Could you check a few things on this model? Use its own coordinates, in mm. A direction names the side the tool comes from. Round coordinates to 2 decimals unless told otherwise and drop trailing zeros. Loops run counter-clockwise (first coordinate to the right, second up) from the corner with the lowest first, then second, coordinate; pieces in that order, holes last. Notation, with made-up numbers: (25.5, -35) -> (65.5, -35) arc R16 cw to (65.5, -9) -> close; hole circle Ø2 at (36.25, -8.5). An arc over 180 degrees is marked (long way). Write each question's results on one line, items separated by ' | '.
Autodesk Inventor part; units mm, degrees
ref_plane "YZ Plane" through (0, 0, 0) normal (1, 0, 0) x (0, 1, 0)
ref_plane "XZ Plane" through (0, 0, 0) normal (0, 1, 0) x (-1, 0, 0)
ref_plane "XY Plane" through (0, 0, 0) normal (0, 0, 1) x (1, 0, 0)
sketch "Sketch1" plane through (0, 0, 0) normal (0, 0, 1) x (1, 0, 0)
  circle A0 centre (0, 0) radius 1.5
  dimension "d0" = 3
extrude "Extrusion1" add sketch "Sketch1" along normal blind 4
sketch "Sketch2" plane through (0, 0, 4) normal (0, 0, 1) x (1, 0, 0)
  circle A0 centre (0, 0) radius 1.5
  circle A1 centre (0, 0) radius 2.5
  dimension "d4" = 5
extrude "Extrusion2" add sketch "Sketch2" along normal blind 6 contours A0 | A1
thread "Thread1"
sketch "Sketch3" plane through (0, 0, 10) normal (0, 0, 1) x (1, 0, 0)
  circle A0 centre (0, 0) radius 2.5
  circle A1 centre (0, 0) radius 4
  dimension "d10" = 8
extrude "Extrusion3" add sketch "Sketch3" along normal blind 6 contours A0 | A1
properties part number "5mm Screw"
1) I want a section at D-D, the plane y = -2.25. Write out the boundary of the cut face in (x, z), plus the area to 3 significant figures.
Model answer:
outline: (-3.31, 10) -> (-1.09, 10) -> (-1.09, 4) -> (1.09, 4) -> (1.09, 10) -> (3.31, 10) -> (3.31, 16) -> (-3.31, 16) -> close | area: 52.8 mm2
2) For faces 1 (the cylindrical face through (-0.867, 3.905, 12.958)), 2 (the cylindrical face through (-1.5, -0.07, 1.97)), which set-ups out of +Z, -Z, +X, -X, +Y, -Y let a thin tool reach every point of the face, with its end or its side?
Model answer:
face 1: +Z, -Z | face 2: -Z
3) I want a section at A-A, the plane y = 0. Write out the boundary of the cut face in (x, z), plus the area to 3 significant figures.
Model answer:
outline: (-4, 10) -> (-2.5, 10) -> (-2.5, 4) -> (-1.5, 4) -> (-1.5, 0) -> (1.5, 0) -> (1.5, 4) -> (2.5, 4) -> (2.5, 10) -> (4, 10) -> (4, 16) -> (-4, 16) -> close | area: 90.0 mm2
4) I need wall thicknesses on line 1 (Z direction, x = 1.5, y = -0.75); line 2 (Z direction, x = 2.5, y = -1.25); line 3 (Y direction, x = 0, z = 7.25). Which ranges of each line are inside material? Lowest first, please.
Model answer:
line 1: z = 4 to 16 | line 2: z = 10 to 16 | line 3: y = -2.5 to 2.5
5) I'm going to push flat-ended pins straight in: pin 1 (1 mm diameter, centred on y = 2.5, z = 2, fed in from +X); pin 2 (1 mm diameter, centred on y = -1.5, z = 9, fed in from -X). Where does each tip first touch, or does it pass through?
Model answer:
pin 1: passes through | pin 2: stops at x = -2.29
6) I want a section at C-C, the plane z = 2. Write out the boundary of the cut face in (x, y), plus the area to 3 significant figures.
Model answer:
outline: circle Ø3 at (0, 0) | area: 7.07 mm2
